The listing builds one solid part. Answer for the finished solid, in the listing's coordinates (mm). Give positions to 0.01 mm unless a question says otherwise; leave off trailing zeros. Write each loop counter-clockwise with the first axis right and the second up, starting at its lowest first coordinate (ties: lowest second). Pieces come first, ordered by that corner, then holes. Notation, with made-up numbers: (52.5, 6.25) - (87.5, 6.25) arc R18 ccw to (87.5, 18.25) - close; hole circle Ø4 at (8.25, -29). An arc over 180 degrees is marked (long way). Return JSON: item names as keys, results as strings.
from build123d import *

# Parameters (mm, degrees)
BOSS_EXTRUDE1_DEPTH = 73.1012


with BuildPart() as part:
    # Sketch1 → Boss-Extrude1 (new, symmetric)
    with BuildSketch(Plane(origin=(0, 0, 0), x_dir=(0, 0, -1), z_dir=(1, 0, 0))):
        with BuildLine():
            Line((-225.810623786, -153.325114244), (-224.691047691, -154.450594417))
            ThreePointArc((-224.691047691, -154.450594417), (-119.024013128, -67.811130366), (1.233217804, -2.925713414))
            Line((1.233217804, -2.925713414), (0.616608902, -1.462856707))
            ThreePointArc((0.616608902, -1.462856707), (-119.908343561, -66.492754113), (-225.810623786, -153.325114244))
        make_face()
        with BuildLine():
            Line((-226.93019988, -152.199634071), (-225.810623786, -153.325114244))
            ThreePointArc((-225.810623786, -153.325114244), (-119.908343561, -66.492754113), (0.616608902, -1.462856707))
            Line((0.616608902, -1.462856707), (0, 0))
            ThreePointArc((0, 0), (-120.792673993, -65.17437786), (-226.93019988, -152.199634071))
        make_face()
    extrude(amount=BOSS_EXTRUDE1_DEPTH, both=True)


solid = part.part
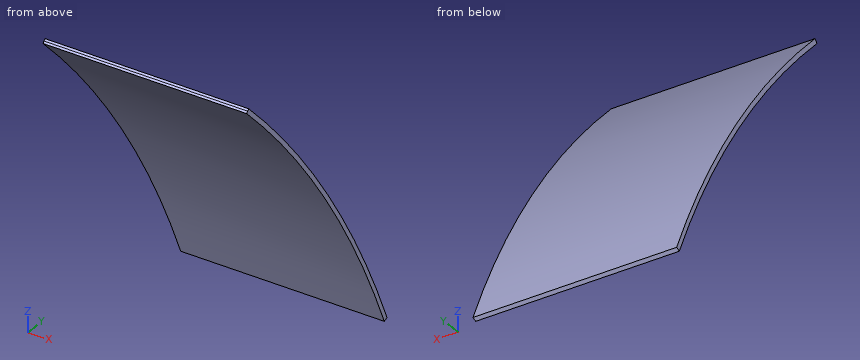
Item 1: A cutting plane is placed at B-B on z = 157.5. Determine the outline of the cut face in (x, y).
Answer below:
{"outline": "(-73.1, -95.52) - (73.1, -95.52) - (73.1, -91.51) - (-73.1, -91.51) - close"}
Item 2: A cutting plane is placed at A-A on x = 47. Determine the outline of the cut face in (y, z), then the cut area to 3 significant figures.
Answer below:
{"outline": "(-154.45, 224.69) arc R712.84 cw to (-2.93, -1.23) - (0, 0) arc R716.01 ccw to (-152.2, 226.93) - close", "area": "871 mm²"}
Item 3: Flat-ended cylindrical pins translate along their axes: P1, Ø5, axis at x = 26.5, y = -123, coming from the -Z side; P2, Ø6, axis at x = -3, z = 184, coming from the +Y side; P3, Ø4, axis at x = 9, y = -112.5, coming from the -Z side. Find the tip coordinate at first contact, or state that the pin passes through.
Answer below:
{"P1": "stops at z = 188.08", "P2": "stops at y = -110.32", "P3": "stops at z = 176.25"}
Item 4: Consider L1, parallel to Y at x = 18, z = 216.5; L2, parallel to Y at x = 29, z = 144.5; L3, parallel to Z at x = 54.5, y = -13. Determine where each line is inside the solid, lowest interval first.
Answer below:
{"L1": "y = -146.43 to -142.03", "L2": "y = -85.72 to -81.78", "L3": "z = 21.55 to 29.03"}
